from build123d import *

# Parameters (mm, degrees)
BOSS_EXTRUDE1_DEPTH          = 10
SKETCH2_W                    = 33.8
SKETCH2_H                    = 18
CUT_EXTRUDE1_DEPTH           = 38
SKETCH3_W                    = 23
SKETCH3_H                    = 40.02
CUT_EXTRUDE2_DEPTH           = 51
CAVITY1_START                = -212
CAVITY1_OUTLINE_W            = 50
CAVITY1_OUTLINE_H            = 10
CAVITY1_DEPTH                = 10
CAVITY1_START_2              = 8
CAVITY1_2_OUTLINE_W          = 50
CAVITY1_2_OUTLINE_H          = 10
CAVITY1_2_DEPTH              = 10
CAVITY1_START_3              = -172
CAVITY1_3_OUTLINE_W          = 10
CAVITY1_3_OUTLINE_H          = 10
CAVITY1_3_DEPTH              = 30
CAVITY1_START_4              = -112
CAVITY1_4_OUTLINE_W          = 10
CAVITY1_4_OUTLINE_H          = 10
CAVITY1_4_DEPTH              = 30
CAVITY1_START_5              = -52
CAVITY1_5_OUTLINE_W          = 10
CAVITY1_5_OUTLINE_H          = 10
CAVITY1_5_DEPTH              = 30
F_3_0_3_DIAMETER_HOLE1_D     = 3
F_3_0_3_DIAMETER_HOLE1_DEPTH = 15
F_3_0_3_DIAMETER_HOLE1_TIP   = 0.901290929


# Read off the part's stored shape, not the designer's step: Cavity1
with BuildPart() as part:
    # Sketch1 → Boss-Extrude1 (new body)
    with BuildSketch(Plane.XY):
        Polygon((18, -35.36), (-12.7, -35.36), (-12.7, 0), (-181.3, 0), (-181.3, -35.36), (-212, -35.36), (-212, -1039.94), (18, -1039.94), align=None)
    extrude(amount=-BOSS_EXTRUDE1_DEPTH)

    # Sketch2 → Cut-Extrude1 (cut)
    with BuildSketch(Plane.XY):
        with Locations((-62.6, -9)):
            Rectangle(SKETCH2_W, SKETCH2_H)
        with Locations((-131.4, -9)):
            Rectangle(SKETCH2_W, SKETCH2_H)
        with Locations((-131.4, -1030.94)):
            Rectangle(SKETCH2_W, SKETCH2_H)
        with Locations((-62.6, -1030.94)):
            Rectangle(SKETCH2_W, SKETCH2_H)
    extrude(amount=-CUT_EXTRUDE1_DEPTH, mode=Mode.SUBTRACT)

    # Sketch3 → Cut-Extrude2 (cut)
    with BuildSketch(Plane.XY):
        with Locations((-200.5, -1019.93)):
            Rectangle(SKETCH3_W, SKETCH3_H)
        with Locations((6.5, -1019.93)):
            Rectangle(SKETCH3_W, SKETCH3_H)
    extrude(amount=-CUT_EXTRUDE2_DEPTH, mode=Mode.SUBTRACT)

    # Cavity1 outline → Cavity1 (cut)
    with BuildSketch(Plane.YZ.offset(CAVITY1_START)):
        with Locations((-110.46, -5)):
            Rectangle(CAVITY1_OUTLINE_W, CAVITY1_OUTLINE_H)
        with Locations((-442.46, -5)):
            Rectangle(CAVITY1_OUTLINE_W, CAVITY1_OUTLINE_H)
        with Locations((-774.46, -5)):
            Rectangle(CAVITY1_OUTLINE_W, CAVITY1_OUTLINE_H)
    extrude(amount=CAVITY1_DEPTH, mode=Mode.SUBTRACT)

    # Cavity1 2 outline → Cavity1 2 (cut)
    with BuildSketch(Plane.YZ.offset(CAVITY1_START_2)):
        with Locations((-442.46, -5)):
            Rectangle(CAVITY1_2_OUTLINE_W, CAVITY1_2_OUTLINE_H)
        with Locations((-774.46, -5)):
            Rectangle(CAVITY1_2_OUTLINE_W, CAVITY1_2_OUTLINE_H)
    extrude(amount=CAVITY1_2_DEPTH, mode=Mode.SUBTRACT)

    # Cavity1 3 outline → Cavity1 3 (cut)
    with BuildSketch(Plane.YZ.offset(CAVITY1_START_3)):
        with Locations((-40.46, -5)):
            Rectangle(CAVITY1_3_OUTLINE_W, CAVITY1_3_OUTLINE_H)
        with Locations((-372.46, -5)):
            Rectangle(CAVITY1_3_OUTLINE_W, CAVITY1_3_OUTLINE_H)
        with Locations((-704.46, -5)):
            Rectangle(CAVITY1_3_OUTLINE_W, CAVITY1_3_OUTLINE_H)
    extrude(amount=CAVITY1_3_DEPTH, mode=Mode.SUBTRACT)

    # Cavity1 4 outline → Cavity1 4 (cut)
    with BuildSketch(Plane.YZ.offset(CAVITY1_START_4)):
        with Locations((-40.46, -5)):
            Rectangle(CAVITY1_4_OUTLINE_W, CAVITY1_4_OUTLINE_H)
        with Locations((-372.46, -5)):
            Rectangle(CAVITY1_4_OUTLINE_W, CAVITY1_4_OUTLINE_H)
        with Locations((-704.46, -5)):
            Rectangle(CAVITY1_4_OUTLINE_W, CAVITY1_4_OUTLINE_H)
    extrude(amount=CAVITY1_4_DEPTH, mode=Mode.SUBTRACT)

    # Cavity1 5 outline → Cavity1 5 (cut)
    with BuildSketch(Plane.YZ.offset(CAVITY1_START_5)):
        with Locations((-40.46, -5)):
            Rectangle(CAVITY1_5_OUTLINE_W, CAVITY1_5_OUTLINE_H)
        with Locations((-372.46, -5)):
            Rectangle(CAVITY1_5_OUTLINE_W, CAVITY1_5_OUTLINE_H)
        with Locations((-704.46, -5)):
            Rectangle(CAVITY1_5_OUTLINE_W, CAVITY1_5_OUTLINE_H)
    extrude(amount=CAVITY1_5_DEPTH, mode=Mode.SUBTRACT)

    # Ø3.0 (3) Diameter Hole1
    with Locations(Plane(origin=(0, 0, -10), x_dir=(-1, 0, 0), z_dir=(0, 0, -1))):
        with Locations((162, -971.94), (32, -68), (162, -68), (32, -971.94), (32, -519.97), (162, -519.97), (97, -1030.94), (168.65, -1030.94), (25.35, -1030.94), (25.35, -9), (168.65, -9), (97, -9)):
            Hole(F_3_0_3_DIAMETER_HOLE1_D / 2, depth=F_3_0_3_DIAMETER_HOLE1_DEPTH)
            with Locations((0, 0, -(F_3_0_3_DIAMETER_HOLE1_DEPTH + F_3_0_3_DIAMETER_HOLE1_TIP / 2))):  # 118° drill point
                Cone(0, F_3_0_3_DIAMETER_HOLE1_D / 2, F_3_0_3_DIAMETER_HOLE1_TIP, mode=Mode.SUBTRACT)


solid = part.part
Can you work these out from the model? Positions are in its coordinate system, mm. Coordinates: 2 decimals unless noted, no trailing zeros. Write each loop counter-clockwise with the first axis right and the second up, starting at its lowest first coordinate (ties: lowest second). Pieces come first, ordered by that corner, then holes. Notation, with made-up numbers: (-20.75, -17.5) -> (-8.75, -17.5) arc R5 ccw to (-8.75, -12.5) -> close; hole circle Ø9 at (16.25, 23). An arc over 180 degrees is marked (long way). Write item = value, one per line.
(1) Imagine slicing it at A-A (z = -8.25). State how many separate pieces and enclosed holes the cut face has, and give its area (3 significant figures).
Verdict:
separate_pieces = 1
enclosed_holes = 21
area = 227,000 mm^2
(2) If I drill on probe 1 along Y at (x, z) = (-97, -2.5); probe 2 along Y at (x, z) = (-150.5, -8.5); probe 3 along Y at (x, z) = (-142.5, -6.25), over which ranges is the centre line in solid material (lowest first)?
Verdict:
probe_1 = -1039.94 to -1032.44, -1029.44 to -709.46, -699.46 to -377.46, -367.46 to -45.46, -35.46 to -10.5, -7.5 to 0
probe_2 = -1039.94 to -709.46, -699.46 to -377.46, -367.46 to -45.46, -35.46 to 0
probe_3 = -1021.94 to -709.46, -699.46 to -377.46, -367.46 to -45.46, -35.46 to -18
(3) Imagine slicing it at B-B (x = -62). Please give me the cut outline in (y, z).
Verdict:
outline = (-1021.94, -10) -> (-18, -10) -> (-18, 0) -> (-1021.94, 0) -> close
(4) For pin 1 (3 mm diameter, centred on x = -205, z = -5.5, fed in from -Y), with a flat end and sliding along its axis, tell me the tip position at first contact or that it passes through.
Verdict:
pin_1 = -999.92
